Part model, mm, in its own coordinate system. A direction names the side the tool comes from. Round coordinates to 2 decimals unless told otherwise and drop trailing zeros. Loops run counter-clockwise (first coordinate to the right, second up) from the corner with the lowest first, then second, coordinate; pieces in that order, holes last.
1) Mould opens along X. For faces 1 (the cylindrical face through (-35.22, 0.81, 39.35)), 2 (the flat face through (-29.5, 6, 19)), 3 (the flat face through (-34, 6, 23)), 4 (the cylindrical face through (-36.93, 0.81, 42.9)) say: +X half, -X half, draft (parallel to the pull), parting line (faces both ways), or undercut.
2) Band-saw the part on A-A, the plane x = -19. Write the cut outline in (y, z).
3) Drop flat-ended pins along their axis: P1, Ø3.5, axis at x = 34.67, z = 40.67, coming from the -Y side; P2, Ø8, axis at x = -28.5, z = -1.5, coming from the +Y side; P3, Ø1.5, axis at y = 6.5, z = 14.5, coming from the +X side. Give the stop position or say it passes through.
4) 3-axis set-ups, long thin cutter, end or side, ignore diameter. For faces 5 (the cylindrical face through (36.9, 0.81, 42.93)), 6 (the flat face through (-34, 6, 15)): which of +Z, -Z, +X, -X, +Y, -Y reach the whole face in a straight line?
5) Probe line 1 (X direction, y = 1, z = -40.67); line 2 (Z direction, x = 34.67, y = 0.5); line 3 (Y direction, x = 23, z = -20.5). List the from-to ranges inside material, lowest first.
6) Band-saw the part on B-B, the plane y = 7.5. Write the cut outline in (x, z), then the cut area to 3 significant figures.
from build123d import *

# Parameters (mm, degrees)
SKETCH1_W                                  = 75
SKETCH1_H                                  = 87
BOSS_EXTRUDE1_DEPTH                        = 1.6
SKETCH2_R                                  = 1.43
CUT_EXTRUDE1_DEPTH                         = 58.45485184
MIRROR1_AT_THE_SECOND_PLANE_COPY_1_SKETC_R = 1.43
MIRROR1_AT_THE_SECOND_PLANE_COPY_1_DEPTH   = 58.45485184
FILLET1_R                                  = 2
SKETCH3_W                                  = 8
SKETCH3_H                                  = 8
BOSS_EXTRUDE2_DEPTH                        = 8


with BuildPart() as part:
    # Sketch1 → Boss-Extrude1 (new body)
    with BuildSketch(Plane(origin=(0, 0, 0), x_dir=(1, 0, 0), z_dir=(0, 1, 0))):
        Rectangle(SKETCH1_W, SKETCH1_H)
    extrude(amount=BOSS_EXTRUDE1_DEPTH)

    # Sketch2 → Cut-Extrude1 (cut, through all)
    with BuildSketch(Plane(origin=(0, 1.6, 0), x_dir=(1, 0, 0), z_dir=(0, 1, 0))):
        with Locations(Location((-34.67, 40.67, 0), (0, 0, 270))):
            Circle(SKETCH2_R)
    cut_extrude1 = extrude(amount=-CUT_EXTRUDE1_DEPTH, mode=Mode.SUBTRACT)

    # Mirror1: Cut-Extrude1 across plane
    add(cut_extrude1.mirror(Plane.XY), mode=Mode.SUBTRACT)

    # Mirror1 at the second plane: Cut-Extrude1 across plane
    add(cut_extrude1.mirror(Plane(origin=(0, 0, 0), x_dir=(0, 0, 1), z_dir=(1, 0, 0))), mode=Mode.SUBTRACT)

    # Mirror1 at the second plane copy 1 sketc → Mirror1 at the second plane copy 1 (cut, through all)
    with BuildSketch(Plane(origin=(0, 1.6, 0), x_dir=(-1, 0, 0), z_dir=(0, 1, 0))):
        with Locations(Location((-34.67, 40.67, 0), (0, 0, 270))):
            Circle(MIRROR1_AT_THE_SECOND_PLANE_COPY_1_SKETC_R)
    extrude(amount=-MIRROR1_AT_THE_SECOND_PLANE_COPY_1_DEPTH, mode=Mode.SUBTRACT)

    # Fillet1
    fillet1_edges = [part.edges().sort_by_distance(p)[0] for p in [
        (-37.5, 0.8, 43.5),
        (-37.5, 0.8, -43.5),
        (37.5, 0.8, -43.5),
        (37.5, 0.8, 43.5),
    ]]
    fillet(fillet1_edges, radius=FILLET1_R)

    # Sketch3 → Boss-Extrude2 (add)
    with BuildSketch(Plane(origin=(0, 1.6, 0), x_dir=(1, 0, 0), z_dir=(0, 1, 0))):
        with Locations((-33.5, -19)):
            Rectangle(SKETCH3_W, SKETCH3_H)
    extrude(amount=BOSS_EXTRUDE2_DEPTH)


solid = part.part
Reported:
1. face 1: undercut
1. face 2: +X half
1. face 3: draft
1. face 4: -X half
2. outline: (0, -43.5) - (1.6, -43.5) - (1.6, 43.5) - (0, 43.5) - close
3. P1: stops at y = 0
3. P2: stops at y = 1.6
3. P3: stops at x = -29.5
4. face 5: +Z, +X, +Y, -Y
4. face 6: -Z, +X, -X, +Y
5. line 1: x = -37.5 to -36.1, -33.24 to 33.24, 36.1 to 37.5
5. line 2: z = -43.5 to -42.1, -39.24 to 39.24, 42.1 to 43.5
5. line 3: y = 0 to 1.6
6. outline: (-37.5, 15) - (-29.5, 15) - (-29.5, 23) - (-37.5, 23) - close
6. area: 64.0 mm2
